```python
from build123d import *

# Parameters (mm, degrees)
F0_W        = 74.2
F0_H        = 48.8
F1_DEPTH    = 2.54
F2_W        = 79.4061459601
F2_H        = 53.7425726652
F2_W_2      = 74.2
F2_H_2      = 48.8
F3_DEPTH    = 20.828
F4_R        = 7.62
F5_T1_DEPTH = 79.1425726652
F5_T3_DEPTH = 104.8061459601


# Not quite as in the source:
# - a fillet or chamfer that OpenCascade refuses, or shapes differently, is made with other operations: its cross-section is extruded or revolved along the edge and cut away or added


with BuildPart() as f1:
    # F0 (on Top) → F1 (new body)
    with BuildSketch(Plane.XY):
        with Locations((0.8302908391, 2.9207762395)):
            Rectangle(F0_W, F0_H)
    extrude(amount=F1_DEPTH)

    # F2 (on face) → F3 (join)
    with BuildSketch(Plane.XY.offset(2.54)):
        with Locations((1.1322144419, 3.0947271734)):
            Rectangle(F2_W, F2_H)
        with Locations((0.8302908391, 2.9207762395)):
            Rectangle(F2_W_2, F2_H_2, mode=Mode.SUBTRACT)
    extrude(amount=-F3_DEPTH)

    # F4
    f4_edges = [f1.edges().sort_by_distance(p)[0] for p in [
        (1.132214, 29.966014, 2.54),
        (-38.570859, 3.094727, 2.54),
        (40.835287, 3.094727, 2.54),
        (1.132214, -23.776559, 2.54),
    ]]
    fillet(f4_edges, radius=F4_R)

    # F5: fillet of radius 5.08 on 4 edges, made by hand

    # F5_s2 → F5_t1 (cut)
    with BuildSketch(Plane.XZ.offset(-42.6660135061)):
        with BuildLine():
            ThreePointArc((40.8352874219, -13.208), (39.3473898704, -16.8001024484), (35.7552874219, -18.288))
            Line((35.7552874219, -18.288), (40.8352874219, -18.288))
            Line((40.8352874219, -18.288), (40.8352874219, -13.208))
        make_face()
        with BuildLine():
            ThreePointArc((-33.4908585382, -18.288), (-37.0829609866, -16.8001024484), (-38.5708585382, -13.208))
            Line((-38.5708585382, -13.208), (-38.5708585382, -18.288))
            Line((-38.5708585382, -18.288), (-33.4908585382, -18.288))
        make_face()
    extrude(amount=F5_T1_DEPTH, mode=Mode.SUBTRACT)

    # F5_s4 → F5_t3 (cut)
    with BuildSketch(Plane.YZ.offset(-51.2708585382)):
        with BuildLine():
            ThreePointArc((-18.6965591592, -18.288), (-22.2886616076, -16.8001024484), (-23.7765591592, -13.208))
            Line((-23.7765591592, -13.208), (-23.7765591592, -18.288))
            Line((-23.7765591592, -18.288), (-18.6965591592, -18.288))
        make_face()
        with BuildLine():
            ThreePointArc((29.9660135061, -13.208), (28.4781159545, -16.8001024484), (24.8860135061, -18.288))
            Line((24.8860135061, -18.288), (29.9660135061, -18.288))
            Line((29.9660135061, -18.288), (29.9660135061, -13.208))
        make_face()
    extrude(amount=F5_T3_DEPTH, mode=Mode.SUBTRACT)


solid = f1.part
```
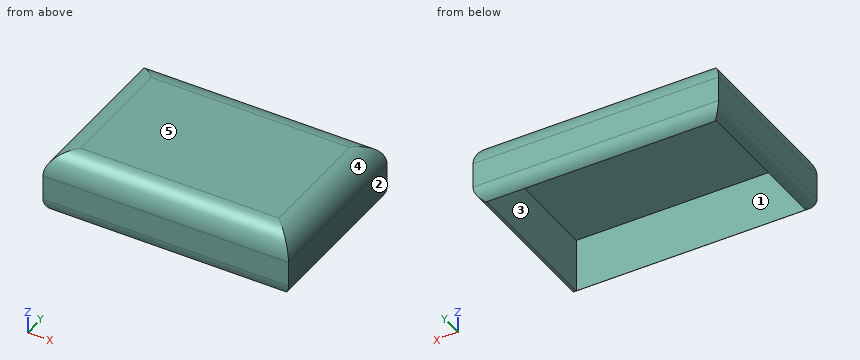
Check sheet for the modelled part. Datum: model origin and axes. Units: mm. Face numbers are marked on the shaded views. A direction names the side the tool comes from. Give positions to 0.01 mm unless a question says otherwise; leave off trailing zeros. Order: outer loops, then holes, each group sorted by start corner. A loop starts at its lowest first (then second) coordinate and runs counter-clockwise, first axis right, second up. Notation, with made-up numbers: (52.25, 48.5) -> (107.25, 48.5) arc R23 ccw to (107.25, 74.5) -> close; hole circle Ø7 at (71.25, 32). An arc over 180 degrees is marked (long way). Use CSV: the item, a comma, the result in double quotes. Start each with the question number.
1) Go/stop test with flat-tipped pins: P1, Ø8, axis at x = -22.5, y = 1.5, coming from the -Z side; P2, Ø2, axis at y = 22.5, z = -14.5, coming from the +X side. Record where each tip stops, or that it passes through.
2) Sectioned sample at A-A, the plane z = -7. Record the boundary of the cut face in (x, y).
3) Material ranges on line 1 (X direction, y = -17, z = -5.75); line 2 (Y direction, x = 8.5, z = -5); line 3 (Z direction, x = 25, y = 2), recorded low to high. Write a range as from..to.
4) Set-up check for the marked faces 1 and 2: record each of +Z, -Z, +X, -X, +Y, -Y from which the full face is reachable in a straight line by a thin tool's end or side.
5) Sectioned sample at B-B, the plane x = -27.5. Record the boundary of the cut face in (y, z).
6) Mould release check, pull along X, two halves, no side actions. Record for the marked faces 3, 4 and 5: released by +X, released by -X, zero draft, split by the parting line, or undercut.
7) Sectioned sample at C-C, the plane y = 19.5. Record the boundary of the cut face in (x, z).
Recorded:
1,P1,"z = 0"
1,P2,"x = 40.83"
2,outline,"(-38.57, -23.78) -> (40.84, -23.78) -> (40.84, 29.97) -> (-38.57, 29.97) -> close; hole (-36.27, -21.48) -> (37.93, -21.48) -> (37.93, 27.32) -> (-36.27, 27.32) -> close"
3,line 1,"-38.57..-36.27, 37.93..40.84"
3,line 2,"-23.78..-21.48, 27.32..29.97"
3,line 3,"0..2.54"
4,face 1,"-Z"
4,face 2,"+Z, -Z, +X, +Y, -Y"
5,outline,"(-23.78, -13.21) arc R5.08 ccw to (-21.48, -17.46) -> (-21.48, 0) -> (27.32, 0) -> (27.32, -17.67) arc R5.08 ccw to (29.97, -13.21) -> (29.97, -5.08) arc R7.62 ccw to (22.35, 2.54) -> (-16.16, 2.54) arc R7.62 ccw to (-23.78, -5.08) -> close"
6,face 3,"undercut"
6,face 4,"released by +X"
6,face 5,"zero draft"
7,outline,"(-38.57, -13.21) arc R5.08 ccw to (-36.27, -17.46) -> (-36.27, 0) -> (37.93, 0) -> (37.93, -17.8) arc R5.08 ccw to (40.84, -13.21) -> (40.84, -5.08) arc R7.62 ccw to (33.22, 2.54) -> (-30.95, 2.54) arc R7.62 ccw to (-38.57, -5.08) -> close"
